Can you work these out from the model? Positions are in its coordinate system, mm. Face numbers are marked on the shaded views. A direction names the side the tool comes from. Round coordinates to 2 decimals unless told otherwise and drop trailing zeros. Write each loop counter-clockwise with the first axis right and the second up, starting at its lowest first coordinate (ties: lowest second). Pieces come first, ordered by that corner, then holes.
Q1. We'd pull the mould along X, two halves only. Please class the marked faces 3, 4 and 5: +X half, -X half, draft (parallel to the pull), parting line (faces both ways), or undercut.
Q2. If we section it at B-B (z = 7): Please give me the cut outline in (x, y), plus the area to 3 significant figures.
Q3. If we section it at C-C (x = 11): Please give me the cut outline in (y, z).
Q4. If we section it at D-D (y = -2): Please give me the cut outline in (x, z), plus the area to 3 significant figures.
Q5. For the marked faces 1 and 2, which set-ups out of +Z, -Z, +X, -X, +Y, -Y let a thin tool reach every point of the face, with its end or its side?
Q6. Please list where these lines run through material, in increasing order: line 1 along Y through (x, z) = (2.25, 3.5); line 2 along X through (y, z) = (-0.5, 2.75); line 3 along Z through (x, y) = (6.5, -3.5).
Q7. If we section it at A-A (y = 0): Please give me the cut outline in (x, z), plus the area to 3 significant figures.
from build123d import *

# Parameters (mm, degrees)
F0_W     = 14
F0_H     = 2
F1_DEPTH = 4
F2_R     = 2.5
F3_DEPTH = 6
F5_R     = 3.5
F6_DEPTH = 12.7


with BuildPart() as f1:
    # F0 (on Front) → F1 (new body, symmetric)
    with BuildSketch(Plane.XZ):
        with Locations((5.8627421725, 1)):
            Rectangle(F0_W, F0_H)
    extrude(amount=F1_DEPTH, both=True)

    # F2 (on face) → F3 (join)
    with BuildSketch(Plane.XY.offset(2)):
        with Locations((9.3627421725, 0)):
            Circle(F2_R)
        with Locations((2.3627421725, 0)):
            Circle(F2_R)
    extrude(amount=F3_DEPTH)

    # F5 (on mid) → F6 (cut, symmetric)
    with BuildSketch(Plane(origin=(5.8627421725, 0, 0), x_dir=(0, -1, 0), z_dir=(-1, 0, 0))):
        with Locations((0, -2.5)):
            Circle(F5_R)
    extrude(amount=F6_DEPTH, both=True, mode=Mode.SUBTRACT)


solid = f1.part
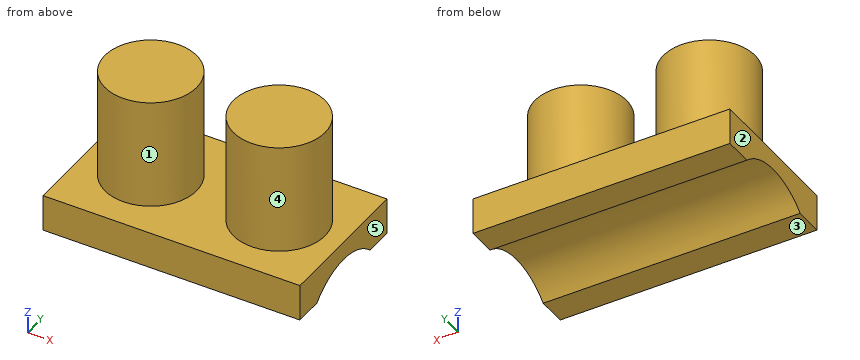
A:
1. face 3: draft
1. face 4: undercut
1. face 5: +X half
2. outline: circle Ø5 at (2.36, 0); circle Ø5 at (9.36, 0)
2. area: 39.3 mm2
3. outline: (-4, 0) - (-2.45, 0) arc R3.5 cw to (2.45, 0) - (4, 0) - (4, 2) - (1.89, 2) - (1.89, 8) - (-1.89, 8) - (-1.89, 2) - (-4, 2) - close
4. outline: (-1.14, 0.37) - (12.86, 0.37) - (12.86, 2) - (10.86, 2) - (10.86, 8) - (7.86, 8) - (7.86, 2) - (3.86, 2) - (3.86, 8) - (0.86, 8) - (0.86, 2) - (-1.14, 2) - close
4. area: 58.8 mm2
5. face 1: +Z
5. face 2: +Z, -Z, -X, +Y, -Y
6. line 1: y = -2.5 to 2.5
6. line 2: x = -0.09 to 4.81, 6.91 to 11.81
6. line 3: z = 0 to 2
7. outline: (-1.14, 1) - (12.86, 1) - (12.86, 2) - (11.86, 2) - (11.86, 8) - (6.86, 8) - (6.86, 2) - (4.86, 2) - (4.86, 8) - (-0.14, 8) - (-0.14, 2) - (-1.14, 2) - close
7. area: 74.0 mm2
